from build123d import *


with BuildPart() as f1:
    # F0 (on Front) → F1 (revolve)
    with BuildSketch(Plane.XZ):
        with BuildLine():
            Line((20.5, 50), (0, 50))
            Line((0, 50), (0, 0))
            Line((0, 0), (45, 0))
            Line((45, 0), (45, 15))
            ThreePointArc((45, 15), (43.535534, 18.535534), (40, 20))
            Line((40, 20), (37, 20))
            ThreePointArc((37, 20), (35.335899, 20.503849), (34.230769, 21.846154))
            Line((34.230769, 21.846154), (23.269231, 48.153846))
            ThreePointArc((23.269231, 48.153846), (22.164101, 49.496151), (20.5, 50))
        make_face()
    revolve(axis=Axis((0, 0, 23.88157), (0, 0, 1)))


solid = f1.part
Design review of the part built by this model. Coordinates are the model's own, in mm. A direction names the side the tool comes from. Give positions to 0.01 mm unless a question says otherwise; leave off trailing zeros. Write each loop counter-clockwise with the first axis right and the second up, starting at its lowest first coordinate (ties: lowest second). Pieces come first, ordered by that corner, then holes. Notation, with made-up numbers: M -27.75,-10 L 19.25,-10 A32 ccw 19.25,26 Z; hole C 70,60.5 d9. An arc over 180 degrees is marked long. Answer as a JSON object with one key per item and string values. Group by question number.
1) We need section A-A (x = 0). Give the boundary of the cut face in (y, z), and give its area (3 significant figures).
2) Tool access review of faces 1 (the face through (11.7, -35.4, 20)), 2 (the face through (20.765, -39.923, 7.605)): name each direction out of +Z, -Z, +X, -X, +Y, -Y from which nothing blocks a thin tool from reaching the whole face with its end or side.
3) For line 1 along Y through (x, z) = (-0.5, 5); line 2 along Z through (x, y) = (27, -27); line 3 along Y through (x, z) = (-22, 11), list the stretches that pass through material, from the lowest coordinate up.
4) We need section D-D (z = 25). Give the boundary of the cut face in (x, y).
5) Clearance check with flat-ended pins moving along their axes: pin 1 Ø12 at (x, y) = (13, -29) entering from +Z; pin 2 Ø12 at (x, y) = (21, 20) entering from +Z; pin 3 Ø12 at (x, z) = (12.5, 23) entering from -Y. State where each tip first meets the part, or that it passes through.
6) We need section C-C (z = 12). Give the boundary of the cut face in (x, y), and give its area (3 significant figures).
Answer key:
{
 "1": {"outline": "M -45,0 L 45,0 L 45,15 A5 ccw 40,20 L 37,20 A3 cw 34.23,21.85 L 23.27,48.15 A3 ccw 20.5,50 L -20.5,50 A3 ccw -23.27,48.15 L -34.23,21.85 A3 cw -37,20 L -40,20 A5 ccw -45,15 Z", "area": "3,510 mm²"},
 "2": {"face 1": "+Z", "face 2": "+Z, -Z"},
 "3": {"line 1": "y = -45 to 45", "line 2": "z = 0 to 20", "line 3": "y = -39.26 to 39.26"},
 "4": {"outline": "C 0,0 d65.83"},
 "5": {"pin 1": "stops at z = 42.13", "pin 2": "stops at z = 48.66", "pin 3": "stops at y = -43.17"},
 "6": {"outline": "C 0,0 d90", "area": "6,360 mm²"}
}
